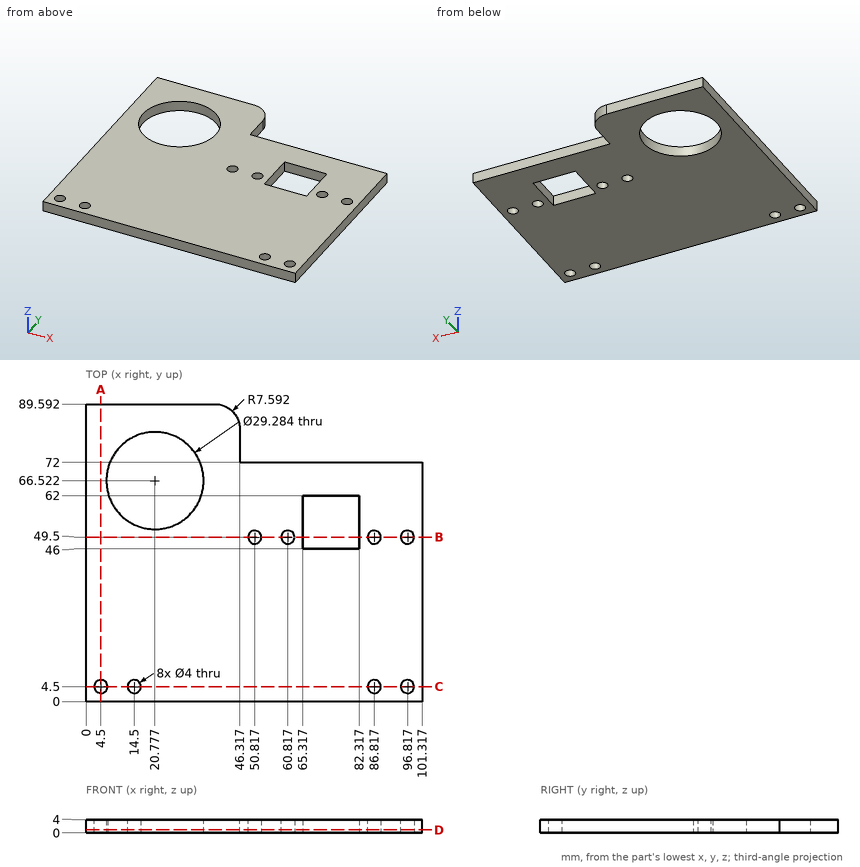
Part print with two shaded views. Sizes in mm from the minimum x, y, z corner. Coordinates: 2 decimals unless noted, no trailing zeros. Write each loop counter-clockwise with the first axis right and the second up, starting at its lowest first coordinate (ties: lowest second). Pieces come first, ordered by that corner, then holes.
1. Drill centre lines: probe 1 along Y at (x, z) = (79, 1.7); probe 2 along Y at (x, z) = (4.5, 1.65); probe 3 along X at (y, z) = (67, 2.1). Where is each one in solid material? Low to high.
Answer block:
probe 1: y = 0 to 46, 62 to 72
probe 2: y = 0 to 2.5, 6.5 to 89.59
probe 3: x = 0 to 6.14, 35.41 to 101.32
2. Band-saw the part on D-D, the plane z = 0.9. Give the number of separate pieces and of enclosed holes in the cut face, and give its area (3 significant figures).
Answer block:
separate pieces: 1
enclosed holes: 10
area: 7,050 mm2
3. Band-saw the part on B-B, the plane y = 49.5. Give the cut face in (x, z).
Answer block:
outline: (0, 0) - (48.82, 0) - (48.82, 4) - (0, 4) - close; (52.82, 0) - (58.82, 0) - (58.82, 4) - (52.82, 4) - close; (62.82, 0) - (65.32, 0) - (65.32, 4) - (62.82, 4) - close; (82.32, 0) - (84.82, 0) - (84.82, 4) - (82.32, 4) - close; (88.82, 0) - (94.82, 0) - (94.82, 4) - (88.82, 4) - close; (98.82, 0) - (101.32, 0) - (101.32, 4) - (98.82, 4) - close
4. Band-saw the part on C-C, the plane y = 4.5. Give the cut face in (x, z).
Answer block:
outline: (0, 0) - (2.5, 0) - (2.5, 4) - (0, 4) - close; (6.5, 0) - (12.5, 0) - (12.5, 4) - (6.5, 4) - close; (16.5, 0) - (84.82, 0) - (84.82, 4) - (16.5, 4) - close; (88.82, 0) - (94.82, 0) - (94.82, 4) - (88.82, 4) - close; (98.82, 0) - (101.32, 0) - (101.32, 4) - (98.82, 4) - close
5. Drop flat-ended pins along their axis: pin 1 (2.5 mm diameter, centred on x = 96.82, y = 49.5, fed in from -Z); pin 2 (1.2 mm diameter, centred on x = 80, z = 1, fed in from +Y); pin 3 (1.2 mm diameter, centred on y = 74.5, z = 2.5, fed in from +X). Give the stop position or say it passes through.
Answer block:
pin 1: passes through
pin 2: stops at y = 72
pin 3: stops at x = 46.32
6. Band-saw the part on A-A, the plane x = 4.5. Give the cut face in (y, z).
Answer block:
outline: (0, 0) - (2.5, 0) - (2.5, 4) - (0, 4) - close; (6.5, 0) - (89.59, 0) - (89.59, 4) - (6.5, 4) - close
